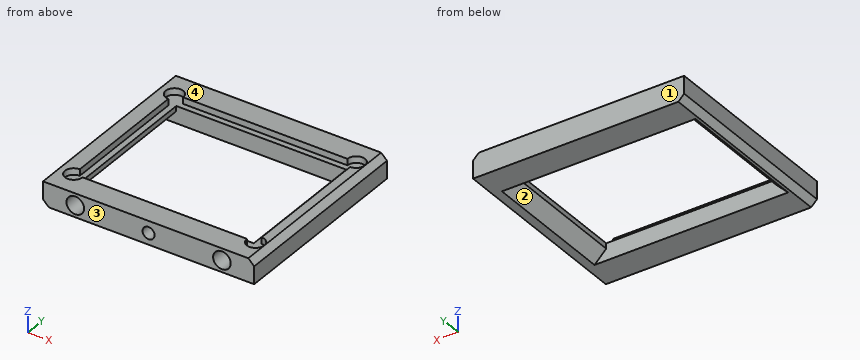
from build123d import *

# Parameters (mm, degrees)
SKETCH1_W                 = 36
SKETCH1_H                 = 33
BOSS_EXTRUDE1_DEPTH       = 4
SKETCH2_W                 = 31
SKETCH2_H                 = 25
CUT_EXTRUDE1_DEPTH        = 1.1
F_3_0MM_DOWEL_HOLE1_D     = 3
F_3_0MM_DOWEL_HOLE1_DEPTH = 1.1
SKETCH5_W                 = 29
SKETCH5_H                 = 23
CUT_EXTRUDE2_DEPTH        = 25.589835298
CHAMFER1_SIZE             = 2
CHAMFER2_SIZE             = 1
F_3_0MM_DOWEL_HOLE2_D     = 3
F_3_0MM_DOWEL_HOLE2_DEPTH = 3.5
F_3_0MM_DOWEL_HOLE2_TIP   = 0.901290929


# Read off the part's stored shape, not the designer's step: M2.5x0.45 Tapped Hole1
with BuildPart() as part:
    # Sketch1 → Boss-Extrude1 (new body)
    with BuildSketch(Plane.XY):
        Rectangle(SKETCH1_W, SKETCH1_H)
    extrude(amount=BOSS_EXTRUDE1_DEPTH)

    # Sketch2 → Cut-Extrude1 (cut)
    with BuildSketch(Plane.XY.offset(4)):
        Rectangle(SKETCH2_W, SKETCH2_H)
    extrude(amount=-CUT_EXTRUDE1_DEPTH, mode=Mode.SUBTRACT)

    # Ø3.0mm Dowel Hole1
    with Locations(Plane.XY.offset(4)):
        with Locations((-15.5, 12.5), (15.5, 12.5), (15.5, -12.5), (-15.5, -12.5)):
            Hole(F_3_0MM_DOWEL_HOLE1_D / 2, depth=F_3_0MM_DOWEL_HOLE1_DEPTH)

    # Sketch5 → Cut-Extrude2 (cut, through all)
    with BuildSketch(Plane.XY.offset(2.9)):
        Rectangle(SKETCH5_W, SKETCH5_H)
    extrude(amount=-CUT_EXTRUDE2_DEPTH, mode=Mode.SUBTRACT)

    # Chamfer1
    chamfer1_edges = [part.edges().sort_by_distance(p)[0] for p in [
        (14.5, 0, 0),
        (-14.5, 0, 0),
    ]]
    chamfer(chamfer1_edges, length=CHAMFER1_SIZE)

    # Chamfer2
    chamfer2_edges = [part.edges().sort_by_distance(p)[0] for p in [
        (18, 0, 4),
        (-18, 0, 0),
    ]]
    chamfer(chamfer2_edges, length=CHAMFER2_SIZE - 0.0001)  # a hair under: the kernel refuses the full size

    # Ø3.0mm Dowel Hole2
    with Locations(Plane(origin=(0, -16.5, 0), x_dir=(-1, 0, 0), z_dir=(0, -1, 0))):
        with Locations((12.5, -2), (-12.5, -2)):
            Hole(F_3_0MM_DOWEL_HOLE2_D / 2, depth=F_3_0MM_DOWEL_HOLE2_DEPTH)
            with Locations((0, 0, -(F_3_0MM_DOWEL_HOLE2_DEPTH + F_3_0MM_DOWEL_HOLE2_TIP / 2))):  # 118° drill point
                Cone(0, F_3_0MM_DOWEL_HOLE2_D / 2, F_3_0MM_DOWEL_HOLE2_TIP, mode=Mode.SUBTRACT)

    # M2.5x0.45 Tapped Hole1 outline → M2.5x0.45 Tapped Hole1 (revolve, cut)
    with BuildSketch(Plane.XY.offset(1.951410637)):
        Polygon((1.025, -13), (0, -12.384117865), (0, -16.5), (1.025, -16.5), align=None)
    revolve(axis=Axis((0, 0, 1.951410637), (0, 1, 0)), mode=Mode.SUBTRACT)


solid = part.part
The model under review builds one solid part; all positions refer to its coordinate system, in mm. Face numbers are marked on the shaded views. Round coordinates to 2 decimals unless told otherwise and drop trailing zeros. Loops run counter-clockwise (first coordinate to the right, second up) from the corner with the lowest first, then second, coordinate; pieces in that order, holes last. Notation, with made-up numbers: (82.25, -1) -> (131.25, -1) arc R28 ccw to (131.25, 29) -> close; hole circle Ø6 at (39.25, 89). An arc over 180 degrees is marked (long way). Answer as CSV lines item,"result".
1) Add section D-D on y = 13. Write out the cut boundary in (x, z), plus the area to 3 significant figures.
Geometry results:
outline,"(-18, 1) -> (-17, 0) -> (18, 0) -> (18, 3) -> (17, 4) -> (16.91, 4) -> (16.91, 2.9) -> (14.09, 2.9) -> (14.09, 4) -> (-14.09, 4) -> (-14.09, 2.9) -> (-16.91, 2.9) -> (-16.91, 4) -> (-18, 4) -> close"
area,"137 mm²"
2) For P1, Ø5, axis at x = -15.5, y = 12.5, coming from the +Z side, flat-tipped, find the tip position at first contact; note if it passes through.
Geometry results:
P1,"stops at z = 4"
3) Add section B-B on x = 5.5. Write out the cut boundary in (y, z), plus the area to 3 significant figures.
Geometry results:
outline,"(-16.5, 0) -> (-11.5, 0) -> (-11.5, 2.9) -> (-12.5, 2.9) -> (-12.5, 4) -> (-16.5, 4) -> close; (11.5, 0) -> (16.5, 0) -> (16.5, 4) -> (12.5, 4) -> (12.5, 2.9) -> (11.5, 2.9) -> close"
area,"37.8 mm²"
4) Add section A-A on y = -8.5. Write out the cut boundary in (x, z), plus the area to 3 significant figures.
Geometry results:
outline,"(-18, 1) -> (-17, 0) -> (-16.5, 0) -> (-14.5, 2) -> (-14.5, 2.9) -> (-15.5, 2.9) -> (-15.5, 4) -> (-18, 4) -> close; (14.5, 2) -> (16.5, 0) -> (18, 0) -> (18, 3) -> (17, 4) -> (15.5, 4) -> (15.5, 2.9) -> (14.5, 2.9) -> close"
area,"20.8 mm²"
5) Add section C-C on x = 15. Write out the cut boundary in (y, z), plus the area to 3 significant figures.
Geometry results:
outline,"(-16.5, 0) -> (-11.5, 0) -> (-11.5, 1.5) -> (11.5, 1.5) -> (11.5, 0) -> (16.5, 0) -> (16.5, 4) -> (13.91, 4) -> (13.91, 2.9) -> (-13.91, 2.9) -> (-13.91, 4) -> (-16.5, 4) -> close"
area,"66.9 mm²"
6) To check wall thickness, follow line 1 along Y through (x, z) = (4, 1.6); line 2 along Y through (x, z) = (-6, 3.2); line 3 along Z through (x, y) = (12.5, -13.9). State the ranges of each line that lie inside material, in increasing order. Write a range as from..to.
Geometry results:
line 1,"y = -16.5..-11.5, 11.5..16.5"
line 2,"y = -16.5..-12.5, 12.5..16.5"
line 3,"z = 0..0.5, 3.5..4"
7) Draft analysis for pull direction Y (two halves, no side actions). For the marked faces 1, 2, 3 and 4, state which applies: pulls with the +Y half, pulls with the -Y half, needs draft (parallel to the pull), parting line crosses it, or undercut.
Geometry results:
face 1,"pulls with the +Y half"
face 2,"undercut"
face 3,"pulls with the -Y half"
face 4,"needs draft"
